```python
from build123d import *

# Parameters (mm, degrees)
F0_R     = 35.1918039157
F0_R_2   = 32.1953483685
F1_DEPTH = 76.2
F2_R     = 32.3619663376
F3_DEPTH = 25.4
F4_DEPTH = 20.32


# Not quite as in the source:
# - a fillet or chamfer that OpenCascade refuses, or shapes differently, is made with other operations: its cross-section is extruded or revolved along the edge and cut away or added


with BuildPart() as f1:
    # F0 (on Top) → F1 (new body)
    with BuildSketch(Plane.XY):
        Circle(F0_R)
        Circle(F0_R_2, mode=Mode.SUBTRACT)
    extrude(amount=F1_DEPTH)

    # F2 (on Top) → F3 (join)
    with BuildSketch(Plane.XY):
        Circle(F2_R)
    extrude(amount=F3_DEPTH)

    # F4 (cut): a face of the model
    f4_faces = [f1.faces().sort_by_distance(p)[0] for p in [
        (0, 0, 25.4),
    ]]
    extrude(f4_faces, amount=-F4_DEPTH, mode=Mode.SUBTRACT)

    # F5: fillet of radius 5.08 on 2 edges, made by hand

    # F5_s1 → F5_t2 (revolve, cut)
    with BuildSketch(Plane.XZ):
        with BuildLine():
            ThreePointArc((35.1918039157, 71.5669402644), (34.377410896, 74.3257438258), (32.1953483685, 76.2))
            Line((32.1953483685, 76.2), (32.2370192575, 76.2926611947))
            ThreePointArc((32.2370192575, 76.2926611947), (33.6935761421, 76.3016), (35.1918039157, 76.3016))
            Line((35.1918039157, 76.3016), (35.2934039157, 76.2))
            Line((35.2934039157, 76.2), (35.2934039157, 71.5669402644))
            Line((35.2934039157, 71.5669402644), (35.1918039157, 71.5669402644))
        make_face()
    revolve(axis=Axis((0, 0, 76.2), (0, 0, 1)), mode=Mode.SUBTRACT)

    # F5_s3 → F5_t4 (revolve, cut)
    with BuildSketch(Plane.XZ):
        with BuildLine():
            ThreePointArc((35.1918039157, 5.08), (33.7039063642, 1.4878975516), (30.1118039157, 0))
            Line((30.1118039157, 0), (30.1118039157, -0.1016))
            Line((30.1118039157, -0.1016), (35.2934039157, -0.1016))
            Line((35.2934039157, -0.1016), (35.2934039157, 5.08))
            Line((35.2934039157, 5.08), (35.1918039157, 5.08))
        make_face()
    revolve(axis=Axis((0, 0, 0), (0, 0, 1)), mode=Mode.SUBTRACT)


solid = f1.part
```
The model under review builds one solid part; all positions refer to its coordinate system, in mm. Give positions to 0.01 mm unless a question says otherwise; leave off trailing zeros. Write each loop counter-clockwise with the first axis right and the second up, starting at its lowest first coordinate (ties: lowest second). Pieces come first, ordered by that corner, then holes. Notation, with made-up numbers: M -9,9 L 15,9 A12 cw 15,32 Z; hole C -38,81.25 d1. An arc over 180 degrees is marked long. Write item = value, one per line. Start each with the question number.
Q1. Mouldability with a two-part tool opening along X and no side actions: class faces 1 (the face through (-6.98, -31.43, 40.14)), 2 (the face through (0, 0, 5.08)), 3 (the face through (0, 0, 0)), 4 (the face through (-25.94, 23.78, 37.86)) as released by +X, released by -X, zero draft, split by the parting line, or undercut.
Q2. We need section A-A (x = 0). State the section outline as (y, z) points.
Q3. Clearance check with flat-ended pins moving along their axes: pin 1 (5 mm diameter, centred on x = -13, z = 57.5, fed in from -Y); pin 2 (4 mm diameter, centred on y = -15.5, z = 40.5, fed in from -X); pin 3 (10 mm diameter, centred on y = 21.5, z = 36.5, fed in from +X). State where each tip first meets the part, or that it passes through.
Q4. We need section C-C (z = 24). State the section outline as (x, y) points, plus the area to 3 significant figures.
Q5. For line 1 (Y direction, x = 0, z = 38); line 2 (Z direction, x = 3, y = -6); line 3 (Y direction, x = -2, z = 46.5), list the stretches that pass through material, from the lowest coordinate up.
Result set:
q1.face_1 = undercut
q1.face_2 = undercut
q1.face_3 = zero draft
q1.face_4 = split by the parting line
q2.outline = M -35.19,5.08 A5.08 ccw -30.11,0 L 30.11,0 A5.08 ccw 35.19,5.08 L 35.19,71.57 A5.08 ccw 32.2,76.2 L 32.2,5.08 L -32.2,5.08 L -32.2,76.2 A5.08 ccw -35.19,71.57 Z
q3.pin_1 = -33.59
q3.pin_2 = -32.5
q3.pin_3 = 31.08
q4.outline = C 0,0 d70.38; hole C 0,0 d64.39
q4.area = 634 mm2
q5.line_1 = -35.19 to -32.2, 32.2 to 35.19
q5.line_2 = 0 to 5.08
q5.line_3 = -35.13 to -32.13, 32.13 to 35.13
